Geometry: final body of the model. Coordinates: model frame, mm. A direction names the side the tool comes from. Coordinates: 2 decimals unless noted, no trailing zeros. Write each loop counter-clockwise with the first axis right and the second up, starting at its lowest first coordinate (ties: lowest second). Pieces come first, ordered by that corner, then holes.
Autodesk Inventor part; units mm, degrees
ref_plane "YZ Plane" through (0, 0, 0) normal (1, 0, 0) x (0, 1, 0)
ref_plane "XZ Plane" through (0, 0, 0) normal (0, 1, 0) x (-1, 0, 0)
ref_plane "XY Plane" through (0, 0, 0) normal (0, 0, 1) x (1, 0, 0)
sketch "Sketch1" plane through (0, 0, 0) normal (0, 1, 0) x (-1, 0, 0)
  line L0 (126.3491, 283.4802) -> (-143.6509, 283.4802)
  line L1 (-143.6509, 283.4802) -> (-143.6509, -366.5198)
  line L2 (-143.6509, -366.5198) -> (126.3491, -366.5198)
  line L3 (126.3491, -366.5198) -> (126.3491, 283.4802)
  point P0 (0, 0)
  dimension "d0" = 650
  dimension "d1" = 270
extrude "Extrusion1" add sketch "Sketch1" along normal blind 7
sketch "Sketch2" plane through (0, 0, 0) normal (0, -1, 0) x (1, 0, 0)
  line L0 (-101.3766, -334.6757) -> (-65.0758, -334.6757)
  line L1 (-65.0758, -334.6757) -> (-65.0758, -293.0626)
  line L2 (-65.0758, -293.0626) -> (-101.3766, -293.0626)
  line L3 (-101.3766, -293.0626) -> (-101.3766, -334.6757)
  line L4 (-97.1426, 224.249) -> (-79.8855, 224.249)
  line L5 (-79.8855, 224.249) -> (-79.8855, 190.7676)
  line L6 (-79.8855, 190.7676) -> (-97.1426, 190.7676)
  line L7 (-97.1426, 190.7676) -> (-97.1426, 224.249)
  line L8 (-106.8404, 242.9144) -> (-83.2262, 242.9144)
  line L9 (-83.2262, 242.9144) -> (-83.2262, 210.6642)
  line L10 (-83.2262, 210.6642) -> (-106.8404, 210.6642)
  line L11 (-106.8404, 210.6642) -> (-106.8404, 242.9144)
  point P0 (0, 0)
sketch "Sketch3" plane through (0, 7, 0) normal (0, 1, 0) x (1, 0, 0)
  line L0 (-102.0983, -222.5922) -> (-73.128, -222.5922)
  line L1 (-73.128, -222.5922) -> (-73.128, -260.2535)
  line L2 (-73.128, -260.2535) -> (-102.0983, -260.2535)
  line L3 (-102.0983, -260.2535) -> (-102.0983, -222.5922)
  point P0 (0, 0)
extrude "Extrusion2" add sketch "Sketch3" along normal blind 70 and the other way blind 5
sketch "Sketch4" plane through (0, 7, 0) normal (0, 1, 0) x (1, 0, 0)
  line L0 (123.5415, -260.2535) -> (92.3696, -260.2535)
  line L1 (92.3696, -260.2535) -> (92.3696, -223.4411)
  line L2 (92.3696, -223.4411) -> (123.5415, -223.4411)
  line L3 (123.5415, -223.4411) -> (123.5415, -260.2535)
  point P0 (0, 0)
extrude "Extrusion3" add sketch "Sketch4" along normal blind 70
sketch "Sketch5" plane through (0, 7, 0) normal (0, 1, 0) x (1, 0, 0)
  line L0 (123.5415, 64.5703) -> (92.3696, 64.5703)
  line L1 (92.3696, 64.5703) -> (92.3696, 104.6485)
  line L2 (92.3696, 104.6485) -> (123.5415, 104.6485)
  line L3 (123.5415, 104.6485) -> (123.5415, 64.5703)
  point P0 (0, 0)
extrude "Extrusion4" add sketch "Sketch5" along normal blind 70
sketch "Sketch6" plane through (0, 7, 0) normal (0, 1, 0) x (1, 0, 0)
  line L0 (-70.3594, 62.7891) -> (-102.4219, 62.7891)
  line L1 (-102.4219, 62.7891) -> (-102.4219, 105.5391)
  line L2 (-102.4219, 105.5391) -> (-70.3594, 105.5391)
  line L3 (-70.3594, 105.5391) -> (-70.3594, 62.7891)
  point P0 (0, 0)
extrude "Extrusion5" add sketch "Sketch6" along normal blind 70
sketch "Sketch7" plane through (0, 7, 0) normal (0, 1, 0) x (1, 0, 0)
  line L0 (-102.4219, 342.1053) -> (-70.3594, 342.1053)
  line L1 (-70.3594, 342.1053) -> (-70.3594, 300.246)
  line L2 (-70.3594, 300.246) -> (-102.4219, 300.246)
  line L3 (-102.4219, 300.246) -> (-102.4219, 342.1053)
  point P0 (0, 0)
extrude "Extrusion6" add sketch "Sketch7" along normal blind 70
sketch "Sketch8" plane through (0, 7, 0) normal (0, 1, 0) x (1, 0, 0)
  line L0 (123.5415, 300.5975) -> (89.9566, 300.5975)
  line L1 (89.9566, 300.5975) -> (89.9566, 340.6771)
  line L2 (89.9566, 340.6771) -> (123.5415, 340.6771)
  line L3 (123.5415, 340.6771) -> (123.5415, 300.5975)
  point P0 (0, 0)
extrude "Extrusion7" add sketch "Sketch8" along normal blind 70
sketch "Sketch9" plane through (0, 7, 0) normal (0, 1, 0) x (1, 0, 0)
  line L0 (33.3984, -64.125) -> (-17.3672, -64.125)
  line L1 (-17.3672, -64.125) -> (-17.3672, -114)
  line L2 (-17.3672, -114) -> (33.3984, -114)
  line L3 (33.3984, -114) -> (33.3984, -64.125)
  point P0 (0, 0)
extrude "Extrusion8" add sketch "Sketch9" along normal blind 70
properties part number "cstand"
Item 1: Pull-direction query (Z, two-part tool) for faces 1 (the flat face through (8, 42, 114)), 2 (the flat face through (108, 42, 223.441)), 3 (the flat face through (-102.098, 42, 242)); classes: released by +Z, released by -Z, zero draft, split by the parting line, or undercut.
Derived:
face 1: released by +Z
face 2: undercut
face 3: zero draft
Item 2: Section A-A, the plane y = 61. Output: boundary loops of the cut face in (x, z) (1 decimal), plus the area to 3 significant figures.
Derived:
outline: (-102.4, -342.1) - (-70.4, -342.1) - (-70.4, -300.2) - (-102.4, -300.2) - close; (-102.4, -105.5) - (-70.4, -105.5) - (-70.4, -62.8) - (-102.4, -62.8) - close; (-102.1, 222.6) - (-73.1, 222.6) - (-73.1, 260.3) - (-102.1, 260.3) - close; (-17.4, 64.1) - (33.4, 64.1) - (33.4, 114) - (-17.4, 114) - close; (90, -340.7) - (123.5, -340.7) - (123.5, -300.6) - (90, -300.6) - close; (92.4, -104.6) - (123.5, -104.6) - (123.5, -64.6) - (92.4, -64.6) - close; (92.4, 223.4) - (123.5, 223.4) - (123.5, 260.3) - (92.4, 260.3) - close
area: 10,100 mm2
Item 3: Pin query (flat end, axial travel): pin 1 (12 mm diameter, centred on y = 47, z = -89.5, fed in from -X); pin 2 (16 mm diameter, centred on x = -84.5, y = 57, fed in from +Z); pin 3 (4 mm diameter, centred on x = -2.5, y = 48, fed in from +Z). Return the tip coordinate at first contact, or that it passes through.
Derived:
pin 1: stops at x = -102.42
pin 2: stops at z = 260.25
pin 3: stops at z = 114
Item 4: Set-up query: faces 4 (the flat face through (-86, 42, -62.789)), 5 (the flat face through (92.37, 42, -84)), 6 (the flat face through (123.542, 42, 242)), 7 (the flat face through (-70.359, 42, -84)), 8 (the flat face through (108, 42, -104.648)). Return all of +Z, -Z, +X, -X, +Y, -Y with unobstructed straight access to the full face (end or side cutting, diameter ignored); none if empty.
Derived:
face 4: +X, -X, +Y
face 5: +Z, +Y
face 6: +Z, -Z, +X, +Y
face 7: +Z, -Z, +Y
face 8: +X, +Y
Item 5: Material intervals for probe 1 along Y at (x, z) = (-34, -100.5); probe 2 along X at (y, z) = (18.5, 83.5); probe 3 along Z at (x, y) = (26, 24) (3 decimals), sorted ascending.
Derived:
probe 1: y = 0 to 7
probe 2: x = -17.37 to 33.4
probe 3: z = 64.125 to 114
Item 6: Section D-D, the plane x = -90. Output: boundary loops of the cut face in (y, z).
Derived:
outline: (0, -366.52) - (7, -366.52) - (7, -342.11) - (77, -342.11) - (77, -300.25) - (7, -300.25) - (7, -105.54) - (77, -105.54) - (77, -62.79) - (7, -62.79) - (7, 222.59) - (77, 222.59) - (77, 260.25) - (7, 260.25) - (7, 283.48) - (0, 283.48) - close
Item 7: Section C-C, the plane z = -94. Output: boundary loops of the cut face in (x, y).
Derived:
outline: (-126.35, 0) - (143.65, 0) - (143.65, 7) - (123.54, 7) - (123.54, 77) - (92.37, 77) - (92.37, 7) - (-70.36, 7) - (-70.36, 77) - (-102.42, 77) - (-102.42, 7) - (-126.35, 7) - close
Item 8: Section B-B, the plane x = -4.5. Output: boundary loops of the cut face in (y, z) (3 decimals), plus the area to 3 significant figures.
Derived:
outline: (0, -366.52) - (7, -366.52) - (7, 64.125) - (77, 64.125) - (77, 114) - (7, 114) - (7, 283.48) - (0, 283.48) - close
area: 8,040 mm2
